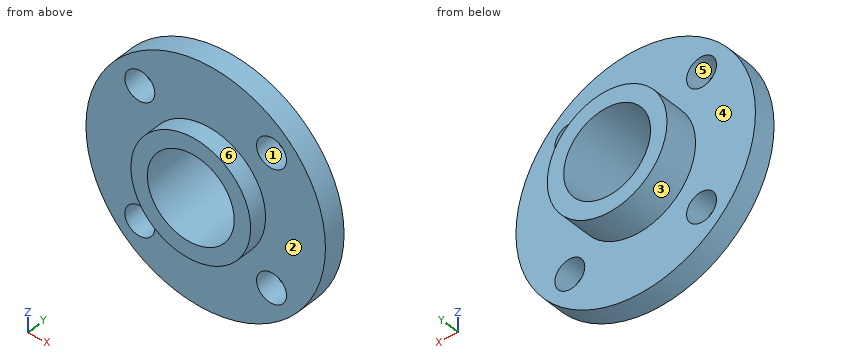
from build123d import *

# Parameters (mm, degrees)
F0_R     = 8
F1_DEPTH = 1.5
F3_D     = 2
F4_R     = 4
F5_DEPTH = 1.2
F6_R     = 4
F7_DEPTH = 2.3
F9_D     = 5.8


with BuildPart() as f1:
    # F0 (on Front) → F1 (new body)
    with BuildSketch(Plane.XZ):
        Circle(F0_R)
    extrude(amount=F1_DEPTH)

    # F3 (through all)
    with Locations(Plane.XZ.offset(1.5)):
        with Locations((-4.4, 4.4), (4.4, 4.4), (4.4, -4.4), (-4.4, -4.4)):
            Hole(F3_D / 2)

    # F4 (on face) → F5 (join)
    with BuildSketch(Plane.XZ.offset(1.5)):
        Circle(F4_R)
    extrude(amount=F5_DEPTH)

    # F6 (on face) → F7 (join)
    with BuildSketch(Plane(origin=(0, 0, 0), x_dir=(-1, 0, 0), z_dir=(0, 1, 0))):
        Circle(F6_R)
    extrude(amount=F7_DEPTH)

    # F9 (through all)
    with Locations(Plane(origin=(0, 2.3, 0), x_dir=(-1, 0, 0), z_dir=(0, 1, 0))):
        with Locations((0, 0)):
            Hole(F9_D / 2)


solid = f1.part
Input: part model. Units: mm. Frame: model coordinates. Face numbers are marked on the shaded views. A direction names the side the tool comes from. Coordinates: 2 decimals unless noted, no trailing zeros. Loops run counter-clockwise (first coordinate to the right, second up) from the corner with the lowest first, then second, coordinate; pieces in that order, holes last. Notation, with made-up numbers: (56, -10.75) -> (85, -10.75) arc R37 cw to (85, 26.25) -> close; hole circle Ø9 at (26, 35). An arc over 180 degrees is marked (long way). One line per item, written item: value.
(1) Cut plane B-B (z = -4.4). Output: boundary loops of the cut face in (x, y).
Answer below:
outline: (-6.68, -1.5) -> (-5.4, -1.5) -> (-5.4, 0) -> (-6.68, 0) -> close; (-3.4, -1.5) -> (3.4, -1.5) -> (3.4, 0) -> (-3.4, 0) -> close; (5.4, -1.5) -> (6.68, -1.5) -> (6.68, 0) -> (5.4, 0) -> close
(2) Set-up query: the marked faces 4, 5 and 6. Return all of +Z, -Z, +X, -X, +Y, -Y with unobstructed straight access to the full face (end or side cutting, diameter ignored); none if empty.
Answer below:
face 4: +Y
face 5: +Y, -Y
face 6: -Y
(3) Ray query, line 1 along Z through (x, y) = (0, -1.6); line 2 along X through (y, z) = (-1.4, -5) (3 decimals). Return the intervals inside material, ascending.
Answer below:
line 1: z = -4 to -2.9, 2.9 to 4
line 2: x = -6.245 to -5.2, -3.6 to 3.6, 5.2 to 6.245
(4) Draft query along Z for the marked faces 1, 2 and 3. Return one class per face: pulls with the +Z half, pulls with the -Z half, needs draft (parallel to the pull), parting line crosses it, or undercut.
Answer below:
face 1: undercut
face 2: needs draft
face 3: parting line crosses it
(5) Cut plane A-A (x = 0). Output: boundary loops of the cut face in (y, z).
Answer below:
outline: (-2.7, -4) -> (-1.5, -4) -> (-1.5, -8) -> (0, -8) -> (0, -4) -> (2.3, -4) -> (2.3, -2.9) -> (-2.7, -2.9) -> close; (-2.7, 2.9) -> (2.3, 2.9) -> (2.3, 4) -> (0, 4) -> (0, 8) -> (-1.5, 8) -> (-1.5, 4) -> (-2.7, 4) -> close
(6) Cut plane D-D (z = 2.5). Output: boundary loops of the cut face in (x, y), then the cut area to 3 significant figures.
Answer below:
outline: (-7.6, -1.5) -> (-3.12, -1.5) -> (-3.12, -2.7) -> (-1.47, -2.7) -> (-1.47, 2.3) -> (-3.12, 2.3) -> (-3.12, 0) -> (-7.6, 0) -> close; (1.47, -2.7) -> (3.12, -2.7) -> (3.12, -1.5) -> (7.6, -1.5) -> (7.6, 0) -> (3.12, 0) -> (3.12, 2.3) -> (1.47, 2.3) -> close
area: 30.0 mm2
(7) Cut plane C-C (y = 0.8). Output: boundary loops of the cut face in (x, z), then the cut area to 3 significant figures.
Answer below:
outline: circle Ø8 at (0, 0); hole circle Ø5.8 at (0, 0)
area: 23.8 mm2
(8) Pin query (flat end, axial travel): pin 1 Ø1.8 at (x, z) = (-4.4, 4.4) entering from -Y; pin 2 Ø3 at (x, z) = (-4.4, -4.4) entering from -Y; pin 3 Ø1 at (x, y) = (-1, -1.5) entering from +Z; pin 4 Ø2 at (x, z) = (-2.5, -5.5) entering from +Y. Return the tip coordinate at first contact, or that it passes through.
Answer below:
pin 1: passes through
pin 2: stops at y = -1.5
pin 3: stops at z = 7.98
pin 4: stops at y = 0
